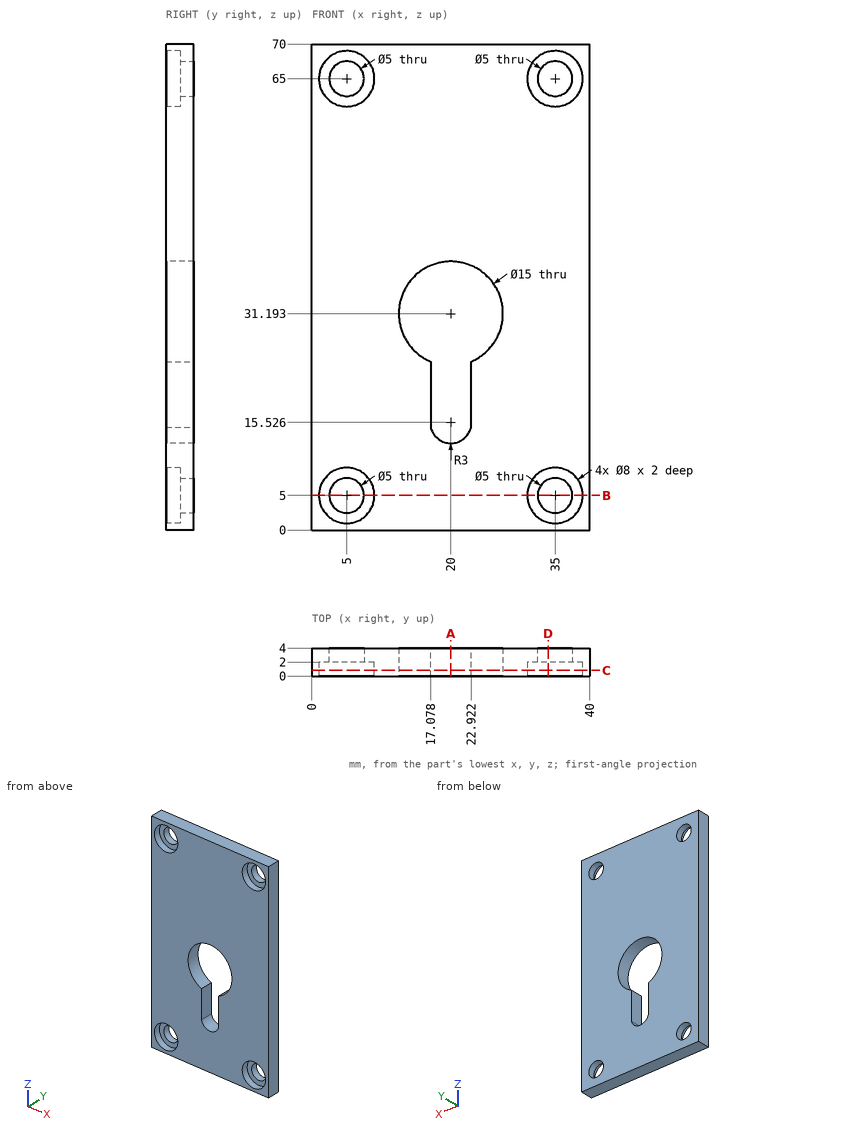
For this review, use the dimensioned drawing (mm, ordinates from the lowest corner) and the shaded views. Round coordinates to 2 decimals unless told otherwise and drop trailing zeros. Write each loop counter-clockwise with the first axis right and the second up, starting at its lowest first coordinate (ties: lowest second). Pieces come first, ordered by that corner, then holes. Notation, with made-up numbers: (68, 10) - (76, 10) arc R31 ccw to (76, 40) - close; hole circle Ø5 at (48.5, 44.5). An arc over 180 degrees is marked (long way). One line per item, written item: value. Start each with the question number.
1. To check wall thickness, follow L1, parallel to Z at x = 5, y = 2.75; L2, parallel to Z at x = 35, y = 0.7; L3, parallel to X at y = 2.3, z = 18.5. State the ranges of each line that lie inside material, in increasing order. Write a range as from..to.
2. Clearance check with flat-ended pins moving along their axes: P1, Ø6.5, axis at x = 35, z = 5, coming from the -Y side; P2, Ø9, axis at x = 36.5, z = 66, coming from the -Y side. State where each tip first meets the part, or that it passes through.
3. Consider section A-A on x = 20. Write out the cut boundary in (y, z), and give its area (3 significant figures).
4. Consider section C-C on y = 0.8. Write out the cut boundary in (x, z), and give its area (3 significant figures).
5. Consider section B-B on z = 5. Write out the cut boundary in (x, y).
6. Consider section D-D on x = 34. Write out the cut boundary in (y, z).
Checks:
1. L1: z = 0..2.5, 7.5..62.5, 67.5..70
1. L2: z = 0..1, 9..61, 69..70
1. L3: x = 0..17.08, 22.92..40
2. P1: stops at y = 2
2. P2: stops at y = 0
3. outline: (0, 0) - (4, 0) - (4, 12.53) - (0, 12.53) - close; (0, 38.69) - (4, 38.69) - (4, 70) - (0, 70) - close
3. area: 175 mm^2
4. outline: (0, 0) - (40, 0) - (40, 70) - (0, 70) - close; hole circle Ø8 at (5, 5); hole circle Ø8 at (5, 65); hole (17.08, 14.85) arc R3 ccw to (22.92, 14.85) - (22.92, 24.29) arc R7.5 ccw (long way) to (17.08, 24.29) - close; hole circle Ø8 at (35, 5); hole circle Ø8 at (35, 65)
4. area: 2,360 mm^2
5. outline: (0, 0) - (1, 0) - (1, 2) - (2.5, 2) - (2.5, 4) - (0, 4) - close; (7.5, 2) - (9, 2) - (9, 0) - (31, 0) - (31, 2) - (32.5, 2) - (32.5, 4) - (7.5, 4) - close; (37.5, 2) - (39, 2) - (39, 0) - (40, 0) - (40, 4) - (37.5, 4) - close
6. outline: (0, 0) - (4, 0) - (4, 2.71) - (2, 2.71) - (2, 1.13) - (0, 1.13) - close; (0, 8.87) - (2, 8.87) - (2, 7.29) - (4, 7.29) - (4, 62.71) - (2, 62.71) - (2, 61.13) - (0, 61.13) - close; (0, 68.87) - (2, 68.87) - (2, 67.29) - (4, 67.29) - (4, 70) - (0, 70) - close
